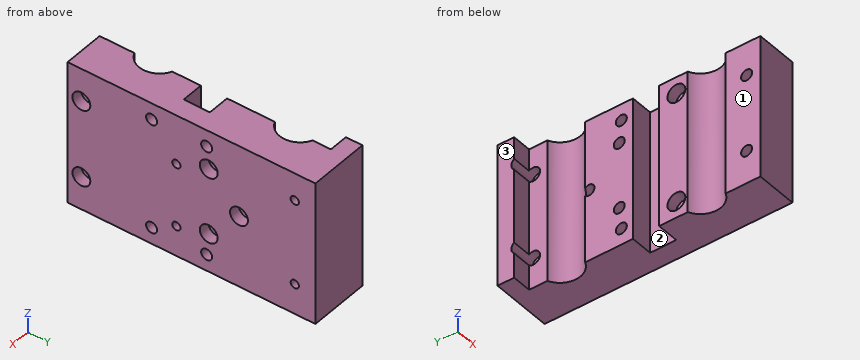
```python
from build123d import *

# Parameters (mm, degrees)
BOSS_EXTRUDE1_DEPTH          = 52
SKETCH2_R                    = 2
CUT_EXTRUDE1_DEPTH           = 100.924971854
ESQUISSE1_R                  = 1.5
ENL_V_MAT_EXTRU_1_DEPTH      = 102.212647431
ENL_V_MAT_EXTRU_2_DEPTH      = 100.924971854
ENL_V_MAT_EXTRU_2_DEPTH_BACK = 3
ESQUISSE2_R                  = 2.5
ESQUISSE3_R                  = 3.25
ENL_V_MAT_EXTRU_3_DEPTH      = 4
ESQUISSE4_R                  = 2
ENL_V_MAT_EXTRU_4_DEPTH      = 102.212647431
ESQUISSE4_3_R                = 3.25
ESQUISSE4_3_R_2              = 2
ENL_V_MAT_EXTRU_5_DEPTH      = 4
ESQUISSE5_R                  = 2
ENL_V_MAT_EXTRU_6_DEPTH      = 100.924971854
ESQUISSE6_R                  = 2
ENL_V_MAT_EXTRU_7_DEPTH      = 102.212647431
ESQUISSE7_R                  = 3.25
ENL_V_MAT_EXTRU_8_DEPTH      = 4
ESQUISSE8_R                  = 7.5
ENL_V_MAT_EXTRU_9_DEPTH      = 100.924971854


with BuildPart() as part:
    # Sketch1 → Boss-Extrude1 (new body)
    with BuildSketch(Plane.XY):
        Polygon((0, 0), (0, -37.75), (8, -37.75), (8, -47.25), (0, -47.25), (0, -84), (15, -84), (15, 6), (-7, 6), (-7, 0), align=None)
    extrude(amount=BOSS_EXTRUDE1_DEPTH)

    # Sketch2 → Cut-Extrude1 (cut, through all)
    with BuildSketch(Plane.ZY):
        with Locations(Location((26, -21.75, 0), (0, 0, 270))):
            Circle(SKETCH2_R)
        with Locations(Location((38, -32.75, 0), (0, 0, 270))):
            Circle(SKETCH2_R)
        with Locations(Location((14, -32.75, 0), (0, 0, 270))):
            Circle(SKETCH2_R)
    extrude(amount=-CUT_EXTRUDE1_DEPTH, mode=Mode.SUBTRACT)

    # Esquisse1 → Enl_v. mat.-Extru.1 (cut, through all)
    with BuildSketch(Plane(origin=(15, 0, 0), x_dir=(0, 0, -1), z_dir=(1, 0, 0))):
        with Locations(Location((-42, -1.5, 0), (0, 0, 90))):
            Circle(ESQUISSE1_R)
        with Locations(Location((-11, -1.5, 0), (0, 0, 90))):
            Circle(ESQUISSE1_R)
        with Locations(Location((-34, -44.5, 0), (0, 0, 90))):
            Circle(ESQUISSE1_R)
        with Locations(Location((-11, -44.5, 0), (0, 0, 90))):
            Circle(ESQUISSE1_R)
    extrude(amount=-ENL_V_MAT_EXTRU_1_DEPTH, mode=Mode.SUBTRACT)

    # Esquisse2 → Enl_v. mat.-Extru.2 (cut, two sides: drawn at the far end of the back side and taken through both)
    with BuildSketch(Plane.ZY.offset(-ENL_V_MAT_EXTRU_2_DEPTH_BACK)):
        with Locations(Location((42, -1.5, 0), (0, 0, 143.130102354))):
            Circle(ESQUISSE2_R)
        with Locations(Location((11, -1.5, 0), (0, 0, 36.869897646))):
            Circle(ESQUISSE2_R)
    extrude(amount=ENL_V_MAT_EXTRU_2_DEPTH + ENL_V_MAT_EXTRU_2_DEPTH_BACK, mode=Mode.SUBTRACT)

    # Esquisse3 → Enl_v. mat.-Extru.3 (cut)
    with BuildSketch(Plane(origin=(15, 0, 0), x_dir=(0, 0, -1), z_dir=(1, 0, 0))):
        with Locations(Location((-26, -21.75, 0), (0, 0, 90))):
            Circle(ESQUISSE3_R)
        with Locations(Location((-14, -32.75, 0), (0, 0, 90))):
            Circle(ESQUISSE3_R)
        with Locations(Location((-38, -32.75, 0), (0, 0, 90))):
            Circle(ESQUISSE3_R)
    extrude(amount=-ENL_V_MAT_EXTRU_3_DEPTH, mode=Mode.SUBTRACT)

    # Esquisse4 → Enl_v. mat.-Extru.4 (cut, through all)
    with BuildSketch(Plane(origin=(15, 0, 0), x_dir=(0, 0, -1), z_dir=(1, 0, 0))):
        with Locations(Location((-40, -79, 0), (0, 0, 90))):
            Circle(ESQUISSE4_R)
        with Locations(Location((-12, -79, 0), (0, 0, 90))):
            Circle(ESQUISSE4_R)
    extrude(amount=-ENL_V_MAT_EXTRU_4_DEPTH, mode=Mode.SUBTRACT)

    # Esquisse4_3 → Enl_v. mat.-Extru.5 (cut)
    # profile 1 of 2: a face of its own
    with BuildSketch(Plane(origin=(15, 0, 0), x_dir=(0, 0, -1), z_dir=(1, 0, 0))):
        with Locations(Location((-12, -79, 0), (0, 0, 90))):
            Circle(ESQUISSE4_3_R)
        with Locations(Location((-12, -79, 0), (0, 0, 90))):
            Circle(ESQUISSE4_3_R_2, mode=Mode.SUBTRACT)
    # profile 2 of 2: a face of its own
    with BuildSketch(Plane(origin=(15, 0, 0), x_dir=(0, 0, -1), z_dir=(1, 0, 0))):
        with Locations(Location((-40, -79, 0), (0, 0, 90))):
            Circle(ESQUISSE4_3_R)
        with Locations(Location((-40, -79, 0), (0, 0, 90))):
            Circle(ESQUISSE4_3_R_2, mode=Mode.SUBTRACT)
    extrude(amount=-ENL_V_MAT_EXTRU_5_DEPTH, mode=Mode.SUBTRACT)

    # Esquisse5 → Enl_v. mat.-Extru.6 (cut, through all)
    with BuildSketch(Plane.ZY):
        with Locations(Location((46, -33.5, 0), (0, 0, 270))):
            Circle(ESQUISSE5_R)
        with Locations(Location((6, -33.5, 0), (0, 0, 270))):
            Circle(ESQUISSE5_R)
    extrude(amount=-ENL_V_MAT_EXTRU_6_DEPTH, mode=Mode.SUBTRACT)

    # Esquisse6 → Enl_v. mat.-Extru.7 (cut, through all)
    with BuildSketch(Plane(origin=(15, 0, 0), x_dir=(0, 0, -1), z_dir=(1, 0, 0))):
        with Locations(Location((-6, -53.5, 0), (0, 0, 90))):
            Circle(ESQUISSE6_R)
        with Locations(Location((-46, -53.5, 0), (0, 0, 90))):
            Circle(ESQUISSE6_R)
    extrude(amount=-ENL_V_MAT_EXTRU_7_DEPTH, mode=Mode.SUBTRACT)

    # Esquisse7 → Enl_v. mat.-Extru.8 (cut)
    with BuildSketch(Plane.ZY):
        with Locations(Location((46, -53.5, 0), (0, 0, 270))):
            Circle(ESQUISSE7_R)
        with Locations(Location((6, -53.5, 0), (0, 0, 270))):
            Circle(ESQUISSE7_R)
    extrude(amount=-ENL_V_MAT_EXTRU_8_DEPTH, mode=Mode.SUBTRACT)

    # Esquisse8 → Enl_v. mat.-Extru.9 (cut, through all)
    with BuildSketch(Plane(origin=(0, 0, 0), x_dir=(-1, 0, 0), z_dir=(0, 0, -1))):
        with Locations((3, -13.5)):
            Circle(ESQUISSE8_R)
        with Locations((3, -64.5)):
            Circle(ESQUISSE8_R)
    extrude(amount=-ENL_V_MAT_EXTRU_9_DEPTH, mode=Mode.SUBTRACT)


solid = part.part
```
For this review, take the finished solid that the model builds, in its own axes (mm). Face numbers are marked on the shaded views. A direction names the side the tool comes from. Give positions to 0.01 mm unless a question says otherwise; leave off trailing zeros. Write each loop counter-clockwise with the first axis right and the second up, starting at its lowest first coordinate (ties: lowest second). Pieces come first, ordered by that corner, then holes. Notation, with made-up numbers: M -38.5,-28 L -2.5,-28 A16 ccw -2.5,-2 Z; hole C -12,24 d11. An arc over 180 degrees is marked long. Answer as a JSON object with one key per item and string values. Group by question number.
Item 1: Tool access review of the marked faces 1, 2 and 3: name each direction out of +Z, -Z, +X, -X, +Y, -Y from which nothing blocks a thin tool from reaching the whole face with its end or side.
Item 2: Consider section C-C on z = 26. Write out the cut boundary in (x, y).
Item 3: Consider section D-D on x = -2.75. Write out the cut boundary in (y, z).
Item 4: Consider section B-B on y = -21.75. Write out the cut boundary in (x, z).
Item 5: For probe 1 along Z at (x, y) = (7.25, -53.5); probe 2 along Z at (x, y) = (8.5, -79); probe 3 along Y at (x, z) = (2.5, 9), list the stretches that pass through material, from the lowest coordinate up. Write a range as [from, to].
Item 6: For pin 1 Ø1.5 at (y, z) = (-31, 23.5) entering from -X; pin 2 Ø5 at (y, z) = (-44.5, 34) entering from -X; pin 3 Ø2 at (y, z) = (-80, 39.5) entering from +X, all flat-tipped, find the tip position at first contact; note any pin that passes through.
Item 7: Consider section A-A on y = -1.5. Write out the cut boundary in (x, z), plus the area to 3 significant figures.
Check result:
{
 "1": {"face 1": "+Z, -Z, -X, -Y", "face 2": "+Z, -Z, -X", "face 3": "+Z, -Z, -X, +Y, -Y"},
 "2": {"outline": "M -7,0 L 0,0 L 0,-6.63 A7.5 cw 1.15,-19.75 L 11,-19.75 L 11,-18.5 L 15,-18.5 L 15,6 L -7,6 Z; M 0,-84 L 15,-84 L 15,-25 L 11,-25 L 11,-23.75 L 0,-23.75 L 0,-37.75 L 8,-37.75 L 8,-47.25 L 0,-47.25 L 0,-57.63 A7.5 cw 0,-71.37 Z"},
 "3": {"outline": "M 0,0 L 6,0 L 6,52 L 0,52 L 0,44 A2.5 cw 0,40 L 0,13 A2.5 cw 0,9 Z"},
 "4": {"outline": "M 0,0 L 15,0 L 15,22.75 L 11,22.75 L 11,24 L 0,24 Z; M 0,28 L 11,28 L 11,29.25 L 15,29.25 L 15,52 L 0,52 Z"},
 "5": {"probe 1": "z = [0, 4], [8, 44], [48, 52]", "probe 2": "z = [0, 10], [14, 38], [42, 52]", "probe 3": "y = [-84, -69.6], [-59.4, -54.75], [-52.25, -47.25], [-37.75, -18.6], [-8.4, -3], [0, 6]"},
 "6": {"pin 1": "stops at x = 0", "pin 2": "stops at x = 8", "pin 3": "stops at x = 11"},
 "7": {"outline": "M 0,0 L 15,0 L 15,9.5 L 3,9.5 L 3,8.5 L 0,8.5 Z; M 0,13.5 L 3,13.5 L 3,12.5 L 15,12.5 L 15,40.5 L 3,40.5 L 3,39.5 L 0,39.5 Z; M 0,44.5 L 3,44.5 L 3,43.5 L 15,43.5 L 15,52 L 0,52 Z", "area": "678 mm^2"}
}
